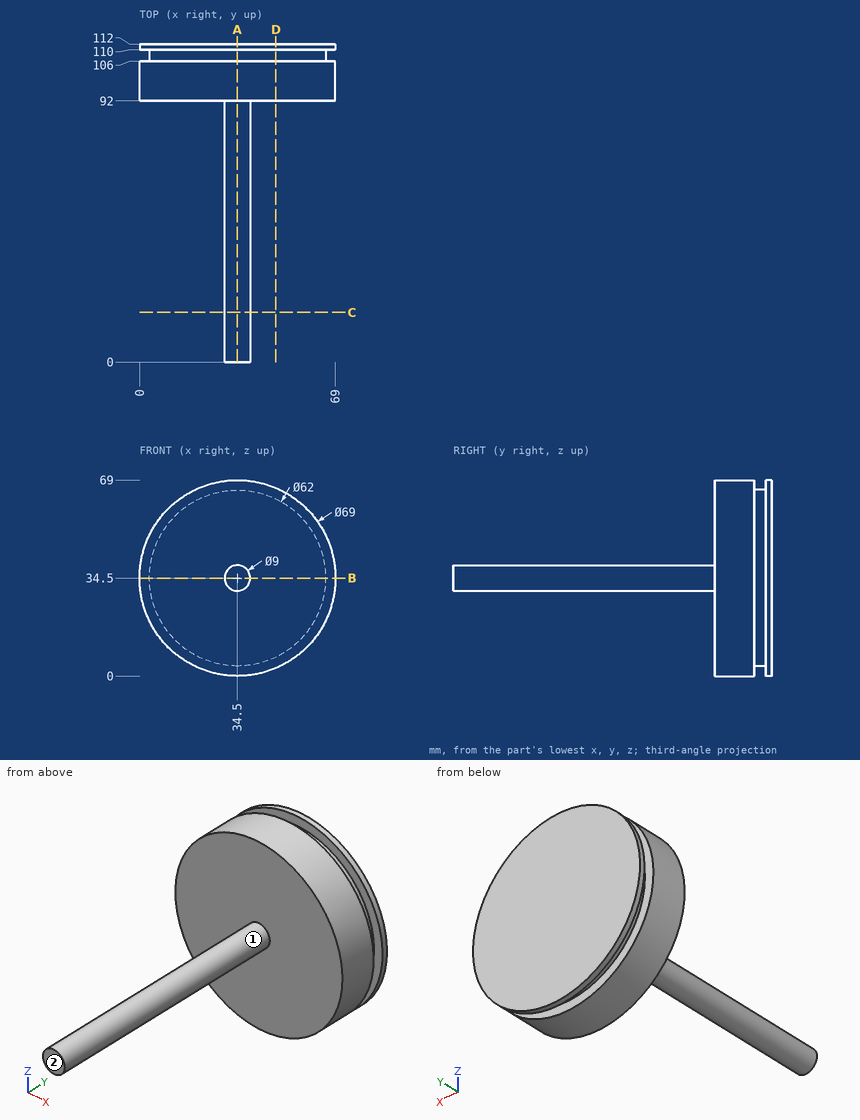
Geometry check sheet. Reference: drawing and pictorial views, mm from the part's lowest x, y, z. A direction names the side the tool comes from. Give positions to 0.01 mm unless a question says otherwise; leave off trailing zeros. Write each loop counter-clockwise with the first axis right and the second up, starting at its lowest first coordinate (ties: lowest second). Pieces come first, ordered by that corner, then holes.
Item 1: Cross-section at B-B (z = 34.5). Enter the section's corners in (x, y), and give its area (3 significant figures).
Item 2: Cross-section at A-A (x = 34.5). Enter the section's corners in (y, z), and give its area (3 significant figures).
Item 3: Gauge pin test, flat ends, axial feed: pin 1 (8 mm diameter, centred on x = 20, z = 29, fed in from -Y); pin 2 (8 mm diameter, centred on y = 35, z = 34.5, fed in from -X); pin 3 (12 mm diameter, centred on x = 36, y = 35, fed in from +Z). Record the tip position at first contact, or that the pin passes through.
Item 4: Cross-section at C-C (y = 17.5). Enter the section's corners in (x, z).
Item 5: Cross-section at D-D (x = 48). Enter the section's corners in (y, z).
Item 6: Access from +Z, -Z, +X, -X, +Y, -Y to the whole of each face (thin tool, end or side, straight path). Record for the marked faces 1 and 2.
Item 7: Scan lines: L1, parallel to Y at x = 43.5, z = 4.5; L2, parallel to Y at x = 9.5, z = 49; L3, parallel to X at y = 105, z = 52. Record each from-to range of solid material in increasing order.
Report:
1. outline: (0, 92) - (30, 92) - (30, 0) - (39, 0) - (39, 92) - (69, 92) - (69, 106) - (65.5, 106) - (65.5, 110) - (69, 110) - (69, 112) - (0, 112) - (0, 110) - (3.5, 110) - (3.5, 106) - (0, 106) - close
1. area: 2,180 mm2
2. outline: (0, 30) - (92, 30) - (92, 0) - (106, 0) - (106, 3.5) - (110, 3.5) - (110, 0) - (112, 0) - (112, 69) - (110, 69) - (110, 65.5) - (106, 65.5) - (106, 69) - (92, 69) - (92, 39) - (0, 39) - close
2. area: 2,180 mm2
3. pin 1: stops at y = 92
3. pin 2: stops at x = 30
3. pin 3: stops at z = 39
4. outline: circle Ø9 at (34.5, 34.5)
5. outline: (92, 2.75) - (106, 2.75) - (106, 6.59) - (110, 6.59) - (110, 2.75) - (112, 2.75) - (112, 66.25) - (110, 66.25) - (110, 62.41) - (106, 62.41) - (106, 66.25) - (92, 66.25) - close
6. face 1: -Y
6. face 2: +Z, -Z, +X, -X, -Y
7. L1: y = 92 to 106, 110 to 112
7. L2: y = 92 to 112
7. L3: x = 4.77 to 64.23
